Autodesk Inventor part; units mm, degrees
ref_plane "XZ Plane" through (0, 0, 0) normal (0, 1, 0) x (-1, 0, 0)
sketch "Sketch1" plane through (0, 0, 0) normal (1, 0, 0) x (0, 1, 0)
  circle A0 centre (0, 0) radius 50
  circle A1 centre (0, 0) radius 62
  dimension "d0" = 100
  dimension "d1" = 124
extrude "Extrusion1" add sketch "Sketch1" along normal blind 30
ref_plane "Work Plane1" through (0, 0, 0) normal (0, 0, 1) x (1, 0, 0)
sketch "Sketch2" plane through (0, 0, 0) normal (0, 0, 1) x (1, 0, 0)
  line L0 (0, 62) -> (30, 62)
  line L1 (18, 62) -> (18, 110)
  line L2 (18, 110) -> (12, 110)
  line L3 (12, 110) -> (12, 62)
  line L4 (0, -62) -> (0, 62)
  line L5 (-6, 0) -> (36, 0)
  point P0 (0, 0)
  dimension "d5" = 6
  dimension "d6" = 12
  dimension "d7" = 48
revolve "Revolution1" add sketch "Sketch2" angle 360 about axis through (-10, 0, 0) along (1, 0, 0)
ref_plane "Work Plane2" through (15, 0, 0) normal (1, 0, 0) x (0, 1, 0)
sketch "Sketch3" plane through (15, 0, 0) normal (1, 0, 0) x (0, 1, 0)
  circle A0 centre (0, 0) radius 130
  circle A1 centre (0, 0) radius 110
  dimension "d10" = 260
  dimension "d11" = 220
extrude "Extrusion2" add sketch "Sketch3" along normal mid plane 25
properties part number "DiscoPaleStadio4-10"
Design review of the part built by this model. Coordinates are the model's own, in mm. A direction names the side the tool comes from. Coordinates: 2 decimals unless noted, no trailing zeros. Loops run counter-clockwise (first coordinate to the right, second up) from the corner with the lowest first, then second, coordinate; pieces in that order, holes last.
Q1. For pin 1 (12 mm diameter, centred on x = 11, y = -26, fed in from +Z); pin 2 (10 mm diameter, centred on y = 24.5, z = -71.5, fed in from -X); pin 3 (10 mm diameter, centred on x = 8.5, y = -45, fed in from +Z), all flat-tipped, find the tip position at first contact; note any pin that passes through.
Reported:
pin 1: stops at z = 128.45
pin 2: stops at x = 12
pin 3: stops at z = 123.69
Q2. We need section A-A on y = 0. State the section outline as (x, z) points, and give its area (3 significant figures).
Reported:
outline: (0, -62) - (12, -62) - (12, -110) - (2.5, -110) - (2.5, -130) - (27.5, -130) - (27.5, -110) - (18, -110) - (18, -62) - (30, -62) - (30, -50) - (0, -50) - close; (0, 50) - (30, 50) - (30, 62) - (18, 62) - (18, 110) - (27.5, 110) - (27.5, 130) - (2.5, 130) - (2.5, 110) - (12, 110) - (12, 62) - (0, 62) - close
area: 2,300 mm2
Q3. Tool access review of faces 1 (the face through (18, 47, -47)), 2 (the face through (5.916, -8.071, -61.472)), 3 (the face through (14.79, 47.69, -15.02)): name each direction out of +Z, -Z, +X, -X, +Y, -Y from which nothing blocks a thin tool from reaching the whole face with its end or side.
Reported:
face 1: +X
face 2: -X
face 3: +X, -X
Q4. We need section C-C on x = 6.25. State the section outline as (y, z) points, and give its area (3 significant figures).
Reported:
outline: circle Ø260 at (0, 0); circle Ø124 at (0, 0); hole circle Ø220 at (0, 0); hole circle Ø100 at (0, 0)
area: 19,300 mm2
Q5. We need section D-D on z = -78.5. State the section outline as (x, y) points, and give its area (3 significant figures).
Reported:
outline: (2.5, -103.62) - (27.5, -103.62) - (27.5, -77.06) - (18, -77.06) - (18, 77.06) - (27.5, 77.06) - (27.5, 103.62) - (2.5, 103.62) - (2.5, 77.06) - (12, 77.06) - (12, -77.06) - (2.5, -77.06) - close
area: 2,250 mm2
Q6. To check wall thickness, follow line 1 (Z direction, x = 24.5, y = 0); line 2 (Y direction, x = 19.25, z = -42); line 3 (X direction, y = -96, z = 13.5). State the ranges of each line that lie inside material, in increasing order.
Reported:
line 1: z = -130 to -110, -62 to -50, 50 to 62, 110 to 130
line 2: y = -123.03 to -101.67, -45.61 to -27.13, 27.13 to 45.61, 101.67 to 123.03
line 3: x = 12 to 18
Q7. The part is to be moulded in two halves that separate along Z. For faces 4 (the face through (15.175, 123.997, 39.048)), 5 (the face through (30, -42, 28)), 6 (the face through (7.316, -23.846, -107.384)), 7 (the face through (22.684, -23.846, 107.384)), say which applies: +Z half, -Z half, draft (parallel to the pull), parting line (faces both ways), or undercut.
Reported:
face 4: parting line
face 5: draft
face 6: undercut
face 7: undercut
